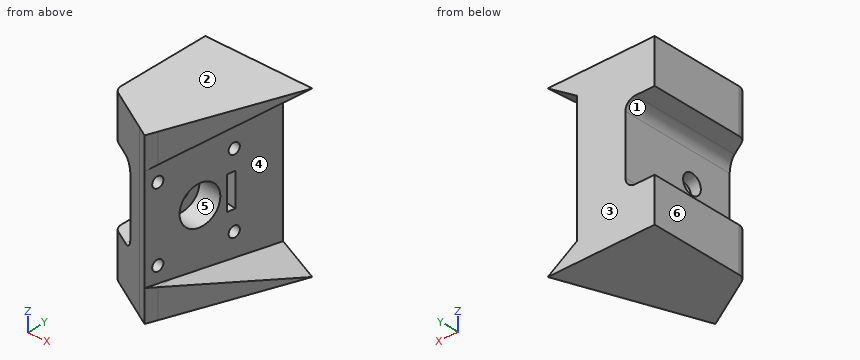
from build123d import *

# Parameters (mm, degrees)
EXTRUDE_1_DEPTH             = 34
CUT_EXTRUDE_1_DEPTH         = 34
CUT_EXTRUDE_12_DEPTH        = 147.490797926
FILLET_1_R                  = 2
CUT_EXTRUDE_13_DEPTH        = 166.02110084
CUT_EXTRUDE_14_DEPTH        = 141.242418962
CUT_EXTRUDE_15_DEPTH        = 141.242418962
EXTRUDE_2_DEPTH             = 34
CUT_EXTRUDE_16_DEPTH        = 141.410480916
EXTRUDE_3_REACH             = 158.273
EXTRUDE_3_DIRECTION_2_REACH = 158.273
SKETCH_24_R                 = 1.1
CUT_EXTRUDE_18_DEPTH        = 3.8
SKETCH_25_RX                = 2
SKETCH_25_RY                = 1.978256004
CUT_EXTRUDE_19_DEPTH        = 8
SKETCH_26_W                 = 6.8
SKETCH_26_H                 = 1.6
CUT_EXTRUDE_20_DEPTH        = 3
SKETCH_27_R                 = 4
SKETCH_27_RX                = 2
SKETCH_27_RY                = 1.978256004
CUT_EXTRUDE_21_DEPTH        = 5


with BuildPart() as part:
    # 草图1 → 凸台-拉伸1 (new body)
    with BuildSketch(Plane.XY):
        with BuildLine():
            Line((111.620742166, -71.457480545), (111.620742166, -52.448586741))
            Line((111.620742166, -52.448586741), (139.548665218, -52.448586741))
            Line((139.548665218, -52.448586741), (129.36488038, -79.948071529))
            ThreePointArc((129.36488038, -79.948071529), (128.178923794, -81.130879534), (126.509316799, -80.996938193))
            Line((126.509316799, -80.996938193), (112.640702972, -73.200903379))
            ThreePointArc((112.640702972, -73.200903379), (111.894463164, -72.467411635), (111.620742166, -71.457480545))
        make_face()
    extrude(amount=EXTRUDE_1_DEPTH)

    # 草图2 → 切除-拉伸1 (cut)
    with BuildSketch(Plane(origin=(0, -52.448586741, 0), x_dir=(1, 0, 0), z_dir=(0, 1, 0))):
        Polygon((129.36488038, -30), (129.36488038, -4), (139.548665218, 0), (139.548665218, -34), align=None)
    extrude(amount=-CUT_EXTRUDE_1_DEPTH, mode=Mode.SUBTRACT)

    # 草图14 → 切除-拉伸12 (cut, through all)
    with BuildSketch(Plane(origin=(0, -52.448586741, 0), x_dir=(1, 0, 0), z_dir=(0, 1, 0))):
        Polygon((111.620742166, -9), (111.620742166, -17), (111.620742166, -25), (117.620742166, -25), (117.620742166, -9), align=None)
    extrude(amount=-CUT_EXTRUDE_12_DEPTH, mode=Mode.SUBTRACT)

    # 圆角1
    fillet_1_edges = [part.edges().sort_by_distance(p)[0] for p in [
        (117.620742166, -64.22447251, 25),
        (117.620742166, -64.22447251, 9),
    ]]
    fillet(fillet_1_edges, radius=FILLET_1_R)

    # 草图15 → 切除-拉伸13 (cut, through all)
    with BuildSketch(Plane.XY.offset(34)):
        with BuildLine():
            Line((129.36488038, -79.948071529), (139.548665218, -52.448586741))
            Line((139.548665218, -52.448586741), (133.548665218, -52.448586741))
            Line((133.548665218, -52.448586741), (124.398706092, -77.156410579))
            ThreePointArc((124.398706092, -77.156410579), (123.212749507, -78.339218585), (121.543142511, -78.205277244))
            Line((121.543142511, -78.205277244), (126.509316799, -80.996938193))
            ThreePointArc((126.509316799, -80.996938193), (128.178923794, -81.130879534), (129.36488038, -79.948071529))
        make_face()
    extrude(amount=-CUT_EXTRUDE_13_DEPTH, mode=Mode.SUBTRACT)

    # 草图16 → 切除-拉伸14 (cut, through all)
    with BuildSketch(Plane(origin=(0, -52.448586741, 0), x_dir=(1, 0, 0), z_dir=(0, 1, 0))):
        Polygon((124.398706092, -5.950620272), (124.398706092, -28.049379728), (129.36488038, -30), (129.36488038, -4), align=None)
    extrude(amount=-CUT_EXTRUDE_14_DEPTH, mode=Mode.SUBTRACT)

    # 草图17 → 切除-拉伸15 (cut, through all)
    with BuildSketch(Plane(origin=(0, -52.448586741, 0), x_dir=(1, 0, 0), z_dir=(0, 1, 0))):
        Polygon((124.398706092, -5.950620272), (124.398706092, -28.049379728), (133.548665218, -34), (133.548665218, 0), align=None)
    extrude(amount=-CUT_EXTRUDE_15_DEPTH, mode=Mode.SUBTRACT)

    # 草图18 → 凸台-拉伸2 (add)
    with BuildSketch(Plane.XY.offset(34)):
        with BuildLine():
            Line((121.543142511, -78.205277244), (123.585184196, -79.353180579))
            Line((123.585184196, -79.353180579), (124.398706092, -77.156410579))
            ThreePointArc((124.398706092, -77.156410579), (123.212749507, -78.339218585), (121.543142511, -78.205277244))
        make_face()
    extrude(amount=-EXTRUDE_2_DEPTH)

    # 草图21 → 切除-拉伸16 (cut, through all)
    with BuildSketch(Plane(origin=(0, -52.448586741, 0), x_dir=(1, 0, 0), z_dir=(0, 1, 0))):
        Polygon((123.585184196, -6.47968929), (123.585184196, -27.52031071), (124.398706092, -28.049379728), (124.398706092, -5.950620272), align=None)
    extrude(amount=-CUT_EXTRUDE_16_DEPTH, mode=Mode.SUBTRACT)

    # 凸台-拉伸3: up to this plane
    extrude_3_end = Plane(origin=(133.548665218, -78.46185441, 34), z_dir=(-0.5451910137179772, 0, 0.8383118504239127))
    # 草图22 → 凸台-拉伸3 (add, up to the surface)
    with BuildSketch(Plane.XY.offset(17), mode=Mode.PRIVATE) as extrude_3_sk1:
        Polygon((127.585184196, -52.448586741), (123.585184196, -79.353180579), (123.585184196, -52.448586741), align=None)
    extrude_3_tool1 = split(extrude(extrude_3_sk1.sketch, amount=EXTRUDE_3_REACH, mode=Mode.PRIVATE), bisect_by=extrude_3_end, keep=Keep.BOTH, mode=Mode.PRIVATE)
    add(extrude_3_tool1.solids().sort_by_distance((124.918518, -61.416785, 17))[0])

    # 凸台-拉伸3 direction 2: up to this plane
    extrude_3_direction_2_end = Plane(origin=(133.548665218, -78.46185441, 0), z_dir=(-0.5451910137179766, 0, -0.838311850423913))
    # 草图22 → 凸台-拉伸3 direction 2 (add, up to the surface)
    with BuildSketch(Plane.XY.offset(17), mode=Mode.PRIVATE) as extrude_3_direction_2_sk1:
        Polygon((127.585184196, -52.448586741), (123.585184196, -79.353180579), (123.585184196, -52.448586741), align=None)
    extrude_3_direction_2_tool1 = split(extrude(extrude_3_direction_2_sk1.sketch, amount=-EXTRUDE_3_DIRECTION_2_REACH, mode=Mode.PRIVATE), bisect_by=extrude_3_direction_2_end, keep=Keep.BOTH, mode=Mode.PRIVATE)
    add(extrude_3_direction_2_tool1.solids().sort_by_distance((124.918518, -61.416785, 17))[0])

    # 草图24 → 切除-拉伸18 (cut)
    with BuildSketch(Plane(origin=(132.455135986, -19.69256801, -116.943153128), x_dir=(0, 0, -1), z_dir=(0.9891280019770362, -0.1470571171515218, 0))):
        with Locations(Location((-141.443153128, -57.716372046, 0), (0, 0, 90))):
            Circle(SKETCH_24_R)
        with Locations(Location((-126.443153128, -57.716372046, 0), (0, 0, 90))):
            Circle(SKETCH_24_R)
        with Locations(Location((-141.443153128, -42.716372046, 0), (0, 0, 90))):
            Circle(SKETCH_24_R)
        with Locations(Location((-126.443153128, -42.716372046, 0), (0, 0, 90))):
            Circle(SKETCH_24_R)
    extrude(amount=-CUT_EXTRUDE_18_DEPTH, mode=Mode.SUBTRACT)

    # 草图25 → 切除-拉伸19 (cut)
    with BuildSketch(Plane(origin=(132.455135986, -19.69256801, -116.943153128), x_dir=(0, 0, -1), z_dir=(0.9891280019770362, -0.1470571171515218, 0))):
        with Locations((-133.943153128, -49.444294674)):
            Ellipse(SKETCH_25_RX, SKETCH_25_RY)
    extrude(amount=-CUT_EXTRUDE_19_DEPTH, mode=Mode.SUBTRACT)

    # 草图26 → 切除-拉伸20 (cut)
    with BuildSketch(Plane(origin=(132.455135986, -19.69256801, -116.943153128), x_dir=(0, 0, -1), z_dir=(0.9891280019770362, -0.1470571171515218, 0))):
        with Locations((-133.943153128, -43.316372046)):
            Rectangle(SKETCH_26_W, SKETCH_26_H)
    extrude(amount=-CUT_EXTRUDE_20_DEPTH, mode=Mode.SUBTRACT)

    # 草图27 → 切除-拉伸21 (cut)
    with BuildSketch(Plane(origin=(132.455135986, -19.69256801, 0), x_dir=(0, 0, -1), z_dir=(0.9891280019770362, -0.1470571171515218, 0))):
        with Locations(Location((-17, -49.444294674, 0), (0, 0, 90))):
            Circle(SKETCH_27_R)
        with Locations((-17, -49.444294674)):
            Ellipse(SKETCH_27_RX, SKETCH_27_RY, mode=Mode.SUBTRACT)
    extrude(amount=-CUT_EXTRUDE_21_DEPTH, mode=Mode.SUBTRACT)


solid = part.part
The listing builds one solid part. Answer for the finished solid, in the listing's coordinates (mm). Face numbers are marked on the shaded views. A direction names the side the tool comes from. Round coordinates to 2 decimals unless told otherwise and drop trailing zeros. Write each loop counter-clockwise with the first axis right and the second up, starting at its lowest first coordinate (ties: lowest second). Pieces come first, ordered by that corner, then holes. Notation, with made-up numbers: (35.5, 81.5) - (52.5, 81.5) arc R15 ccw to (52.5, 88.5) - close; hole circle Ø2 at (85.5, 33.5). An arc over 180 degrees is marked (long way). Use one line per item in the form item = value. Start each with the question number.
Item 1: A cutting plane is placed at B-B (y = -55.25). Write down the section's boundary in (x, z), plus the area to 3 significant figures.
Item 2: A cutting plane is placed at C-C (z = 5.5). Write down the section's boundary in (x, y), plus the area to 3 significant figures.
Item 3: Determine the mould class of the marked faces 3, 4, 5 and 6 for opening direction Y: +Y half, -Y half, draft (parallel to the pull), parting line (faces both ways), or undercut.
Item 4: A tool of negligible diameter and unlimited length cuts with its end or side. For the marked faces 1 and 2, from which of +Z, -Z, +X, -X, +Y, -Y can it reach the whole face along a straight path? Write none if from no direction.
Item 5: A cutting plane is placed at A-A (x = 130.5). Write down the section's boundary in (y, z), plus the area to 3 significant figures.
Item 6: Find the intervals of material crossed by line 1 (Z direction, x = 113.75, y = -65); line 2 (Z direction, x = 124.5, y = -65.25); line 3 (Z direction, x = 124, y = -60.75), in increasing order. Write a range as [from, to].
Item 7: Flat-ended cylindrical pins translate along their axes: pin 1 Ø4 at (x, y) = (118, -61.5) entering from -Z; pin 2 Ø5 at (y, z) = (-69, 24.5) entering from +X; pin 3 Ø2 at (y, z) = (-67, 10.5) entering from -X; pin 4 Ø4 at (x, y) = (129, -72.5) entering from -Z. Find the tip coordinate at first contact, or state that the pin passes through.
Item 8: A cutting plane is placed at D-D (x = 116.5). Write down the section's boundary in (y, z), plus the area to 3 significant figures.
The answers:
q1.outline = (111.62, 0) - (132.51, 0) - (132.51, 0.67) - (127.17, 4.15) - (127.17, 29.85) - (132.51, 33.33) - (132.51, 34) - (111.62, 34) - (111.62, 25) - (115.62, 25) arc R2 cw to (117.62, 23) - (117.62, 11) arc R2 cw to (115.62, 9) - (111.62, 9) - close
q1.area = 460 mm^2
q2.outline = (111.62, -71.46) arc R2 ccw to (112.64, -73.2) - (123.59, -79.35) - (125.09, -75.29) - (125.09, -69.22) - (127.59, -52.45) - (111.62, -52.45) - close
q2.area = 340 mm^2
q3.face_3 = +Y half
q3.face_4 = -Y half
q3.face_5 = undercut
q3.face_6 = draft
q4.face_1 = -X, +Y, -Y
q4.face_2 = +Z, +X, -X, +Y, -Y
q5.outline = (-60.68, 0) - (-52.45, 0) - (-52.45, 1.98) - (-60.68, 1.98) - close; (-60.68, 32.02) - (-52.45, 32.02) - (-52.45, 34) - (-60.68, 34) - close
q5.area = 32.6 mm^2
q6.line_1 = [0, 9], [25, 34]
q6.line_2 = [0, 14.62], [19.38, 34]
q6.line_3 = [0, 8.82], [10.18, 23.82], [25.18, 34]
q7.pin_1 = 0
q7.pin_2 = 125.5
q7.pin_3 = 116.94
q7.pin_4 = through
q8.outline = (-75.37, 0) - (-52.45, 0) - (-52.45, 9.2) - (-75.37, 9.2) - close; (-75.37, 24.8) - (-52.45, 24.8) - (-52.45, 34) - (-75.37, 34) - close
q8.area = 422 mm^2
